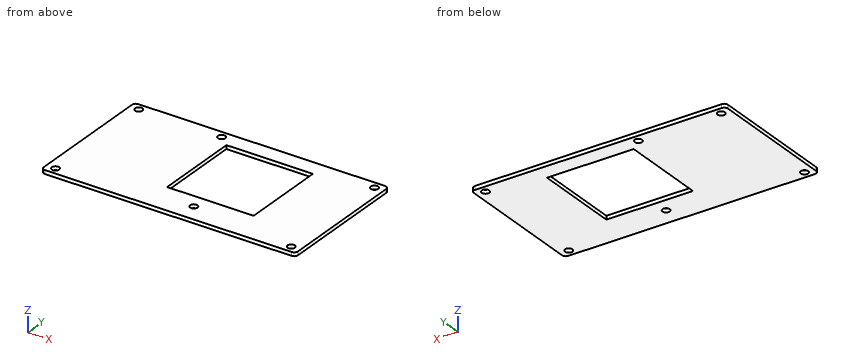
Solid Edge part; units mm, degrees
sketch "Sketch1" plane through (0, 0, 0) normal (0, 0, 1) x (1, 0, 0)
  line L0 (-69, -37) -> (69, -37)
  line L1 (69, -37) -> (69, 37)
  line L2 (69, 37) -> (-69, 37)
  line L3 (-69, 37) -> (-69, -37)
  line L4 (-13, -19) -> (34, -19)
  line L5 (34, -19) -> (34, 28)
  line L6 (34, 28) -> (-13, 28)
  line L7 (-13, 28) -> (-13, -19)
  circle A0 centre (-64, 33) radius 2
  circle A1 centre (-64, -33) radius 2
  circle A2 centre (64, -33) radius 2
  circle A3 centre (7, -27) radius 2
  circle A4 centre (64, 33) radius 2
  circle A5 centre (-19, 33) radius 2
  dimension "D1" = 69
  dimension "D2" = 69
extrude "Protrusion1" add sketch "Sketch1" against normal blind 2
fillet "Congé_1" radius 2 4 edges at (-69, -37, -1) (-69, 37, -1) (69, 37, -1) (69, -37, -1)
Geometry: final body of the model. Coordinates: model frame, mm. Round coordinates to 2 decimals unless told otherwise and drop trailing zeros. Write each loop counter-clockwise with the first axis right and the second up, starting at its lowest first coordinate (ties: lowest second). Pieces come first, ordered by that corner, then holes.
Item 1: Section query D-D (x = -10). Return loops of the section in (y, z), plus the area to 3 significant figures.
Item 2: Section query A-A (x = -64). Return loops of the section in (y, z).
Item 3: Pin query (flat end, axial travel): P1, Ø3, axis at x = -64, y = -33, coming from the -Z side. Return the tip coordinate at first contact, or that it passes through.
Item 4: Section query B-B (z = -1.2). Return loops of the section in (x, y), plus the area to 3 significant figures.
Item 5: Section query C-C (y = -27). Return loops of the section in (x, z).
Item 6: Material intervals for L1, parallel to X at y = 1.5, z = -0.7; L2, parallel to Y at x = -7.5, z = -1.6, sorted ascending.
Completed:
1. outline: (-37, -2) - (-19, -2) - (-19, 0) - (-37, 0) - close; (28, -2) - (37, -2) - (37, 0) - (28, 0) - close
1. area: 54.0 mm2
2. outline: (-37, -2) - (-35, -2) - (-35, 0) - (-37, 0) - close; (-31, -2) - (31, -2) - (31, 0) - (-31, 0) - close; (35, -2) - (37, -2) - (37, 0) - (35, 0) - close
3. P1: passes through
4. outline: (-69, -35) arc R2 ccw to (-67, -37) - (67, -37) arc R2 ccw to (69, -35) - (69, 35) arc R2 ccw to (67, 37) - (-67, 37) arc R2 ccw to (-69, 35) - close; hole circle Ø4 at (-64, -33); hole circle Ø4 at (-64, 33); hole circle Ø4 at (-19, 33); hole (-13, -19) - (34, -19) - (34, 28) - (-13, 28) - close; hole circle Ø4 at (7, -27); hole circle Ø4 at (64, -33); hole circle Ø4 at (64, 33)
4. area: 7,920 mm2
5. outline: (-69, -2) - (5, -2) - (5, 0) - (-69, 0) - close; (9, -2) - (69, -2) - (69, 0) - (9, 0) - close
6. L1: x = -69 to -13, 34 to 69
6. L2: y = -37 to -19, 28 to 37
